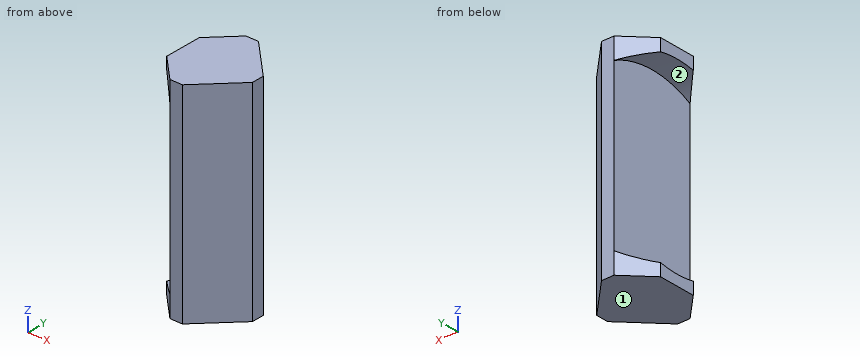
```python
from build123d import *

# Parameters (mm, degrees)
PAD_DEPTH   = 100
SKETCH001_R = 45
HOLE_DEPTH  = 12


with BuildPart() as part:
    # Sketch → Pad (new body)
    with BuildSketch(Plane.XY):
        Polygon((-18, 9), (-18, -9), (-6, -21), (0, -21), (18, -3), (18, 3), (0, 21), (-6, 21), align=None)
    extrude(amount=-PAD_DEPTH)

    # Sketch001 (on Face1 of Pad) → Hole (cut)
    with BuildSketch(Plane(origin=(-18, 0, 0), x_dir=(0, -1, 0), z_dir=(-1, 0, 0))):
        with Locations((0, -50)):
            Circle(SKETCH001_R)
    extrude(amount=-HOLE_DEPTH, mode=Mode.SUBTRACT)


solid = part.part
```
Design review of the part built by this model. Coordinates are the model's own, in mm. Face numbers are marked on the shaded views. A direction names the side the tool comes from. Give positions to 0.01 mm unless a question says otherwise; leave off trailing zeros. Write each loop counter-clockwise with the first axis right and the second up, starting at its lowest first coordinate (ties: lowest second). Pieces come first, ordered by that corner, then holes. Notation, with made-up numbers: (9, 45) -> (50, 45) arc R21 cw to (50, 67) -> close; hole circle Ø9 at (-2, -28.5). An arc over 180 degrees is marked (long way). Answer in a Markdown table with one row per item.
(1) Consider section B-B (x = 4). State the section outline as (y, z) points.
Results:
| item | result |
|---|---|
| outline | (-17, -100) -> (17, -100) -> (17, 0) -> (-17, 0) -> close |
(2) To check wall thickness, follow probe 1 along Z at (x, y) = (-10.5, -0.5); probe 2 along X at (y, z) = (-1.5, -12); probe 3 along Z at (x, y) = (-9.5, -16.5). State the ranges of each line that lie inside material, in increasing order.
Results:
| item | result |
|---|---|
| probe 1 | -100 to -95, -5 to 0 |
| probe 2 | -6 to 18 |
| probe 3 | -100 to -91.87, -8.13 to 0 |
(3) Consider section D-D (y = -17). State the section outline as (x, z) points.
Results:
| item | result |
|---|---|
| outline | (-10, -100) -> (4, -100) -> (4, 0) -> (-10, 0) -> (-10, -8.33) -> (-6, -8.33) -> (-6, -91.67) -> (-10, -91.67) -> close |
(4) Consider section C-C (z = -71.5). State the section outline as (x, y) points, then the cut area to 3 significant figures.
Results:
| item | result |
|---|---|
| outline | (-6, -21) -> (0, -21) -> (18, -3) -> (18, 3) -> (0, 21) -> (-6, 21) -> close |
| area | 684 mm2 |
(5) Consider section A-A (y = 0). State the section outline as (x, z) points.
Results:
| item | result |
|---|---|
| outline | (-18, -100) -> (18, -100) -> (18, 0) -> (-18, 0) -> (-18, -5) -> (-6, -5) -> (-6, -95) -> (-18, -95) -> close |
(6) For the marked faces 1 and 2, list the 3-axis set-ups (+Z, -Z, +X, -X, +Y, -Y) from which the entire face can be reached by the end or side of a thin tool; tool diameter is ignored.
Results:
| item | result |
|---|---|
| face 1 | -Z, +X, -X, +Y, -Y |
| face 2 | -X |
(7) Clearance check with flat-ended pins moving along their axes: pin 1 (10 mm diameter, centred on y = -9.5, z = -78, fed in from +X); pin 2 (8 mm diameter, centred on y = -14.5, z = -18, fed in from -X); pin 3 (10 mm diameter, centred on x = 11, z = -80, fed in from +Y). State where each tip first meets the part, or that it passes through.
Results:
| item | result |
|---|---|
| pin 1 | x = 16.5 |
| pin 2 | x = -6 |
| pin 3 | y = 15 |
